Study the drawing (mm; zero at the part's minimum x, y, z) and answer. A direction names the side the tool comes from. Coordinates: 2 decimals unless noted, no trailing zeros. Order: outer loops, then holes, each group sorted by start corner. A loop starts at its lowest first (then second) coordinate and runs counter-clockwise, first axis right, second up. Notation, with made-up numbers: M 2,20.5 L 40,20.5 A20 cw 40,38.5 Z; hole C -34.75,-18 d2. An arc over 180 degrees is marked long. One line per item, written item: value. Start each with the question number.
Q1. The part is cut by section C-C on z = 0.6. Give the vertices of the cut face in (x, y), then the cut area to 3 significant figures.
Q2. Straight lines are drawn through the part: line 1 along Y through (x, z) = (7.5, 3.55); line 2 along X through (y, z) = (20.55, 3.4); line 3 along Z through (x, y) = (11.75, 22.5). For each, find the intervals that lie inside material, in ascending order. Write a range as [from, to].
Q3. For the marked faces 1, 2 and 3, determine the directions among +Z, -Z, +X, -X, +Y, -Y from which every point of the face is accessible in a straight line to the end or side of a thin tool.
Q4. The part is cut by section A-A on x = 9. Give the vertices of the cut face in (y, z), then the cut area to 4 significant figures.
Q5. Determine the mould class of the marked faces 4, 5 and 6 for opening direction Y: pulls with the +Y half, pulls with the -Y half, needs draft (parallel to the pull), parting line crosses it, or undercut.
Q6. The part is cut by section D-D on y = 20.55. Give the vertices of the cut face in (x, z).
Q7. The part is cut by section B-B on y = 35.5. Give the vertices of the cut face in (x, z).
Q8. Each of these flat-tipped pins is pushed along its axis until it touches: pin 1 Ø0.5 at (y, z) = (5, 1.5) entering from -X; pin 2 Ø3 at (x, y) = (7, 7) entering from -Z; pin 3 Ø5 at (x, y) = (4, 30.5) entering from +Z. Where does it stop, or does it pass through?
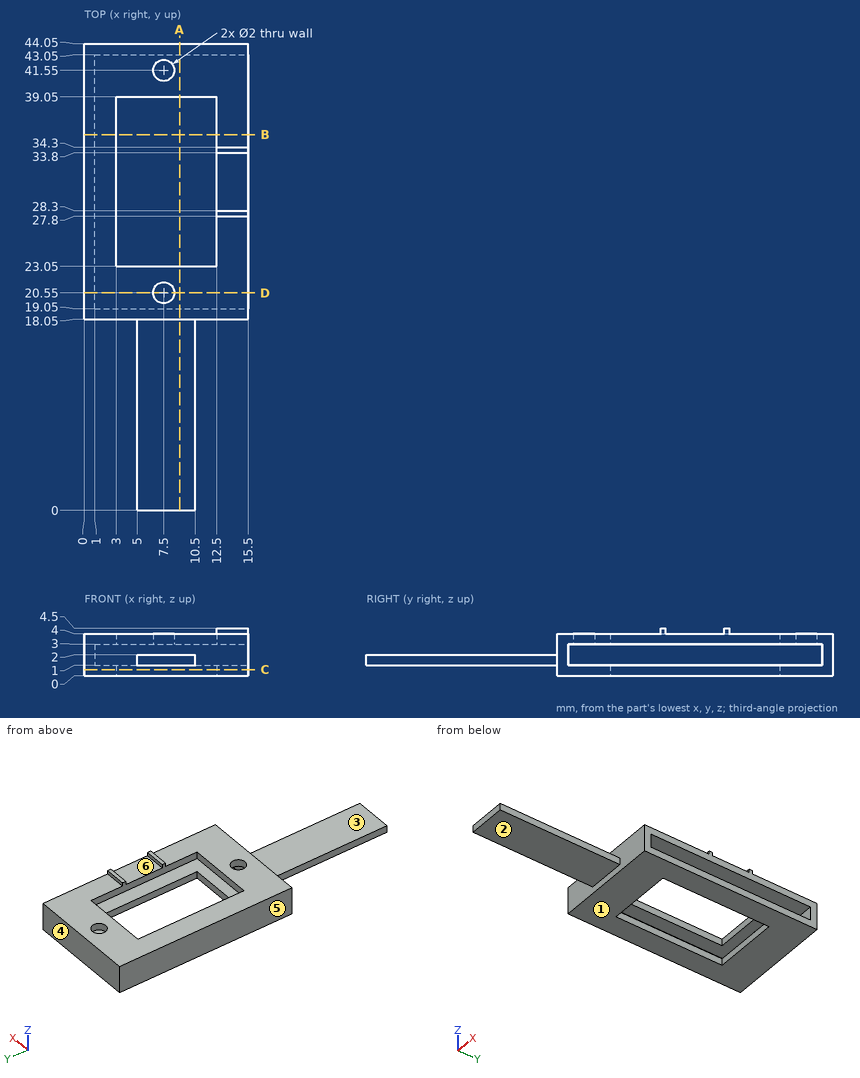
Output:
1. outline: M 0,18.05 L 15.5,18.05 L 15.5,44.05 L 0,44.05 Z; hole M 3,23.05 L 12.5,23.05 L 12.5,39.05 L 3,39.05 Z
1. area: 251 mm^2
2. line 1: y = [18.05, 19.55], [21.55, 23.05], [39.05, 40.55], [42.55, 44.05]
2. line 2: x = [0, 6.5], [8.5, 15.5]
2. line 3: z = [0, 1], [3, 4]
3. face 1: -Z, +X, -X, +Y, -Y
3. face 2: -Z, +X, -X, -Y
3. face 3: +Z, +X, -X, -Y
4. outline: M 0,1 L 18.05,1 L 18.05,0 L 23.05,0 L 23.05,1 L 19.05,1 L 19.05,3 L 23.05,3 L 23.05,4 L 18.05,4 L 18.05,2 L 0,2 Z; M 39.05,0 L 44.05,0 L 44.05,4 L 39.05,4 L 39.05,3 L 43.05,3 L 43.05,1 L 39.05,1 Z
4. area: 42.05 mm^2
5. face 4: pulls with the +Y half
5. face 5: needs draft
5. face 6: undercut
6. outline: M 0,0 L 15.5,0 L 15.5,1 L 1,1 L 1,3 L 6.5,3 L 6.5,4 L 0,4 Z; M 8.5,3 L 15.5,3 L 15.5,4 L 8.5,4 Z
7. outline: M 0,0 L 3,0 L 3,1 L 1,1 L 1,3 L 3,3 L 3,4 L 0,4 Z; M 12.5,0 L 15.5,0 L 15.5,1 L 12.5,1 Z; M 12.5,3 L 15.5,3 L 15.5,4 L 12.5,4 Z
8. pin 1: stops at x = 5
8. pin 2: stops at z = 1
8. pin 3: stops at z = 4
